from build123d import *

# Parameters (mm, degrees)
F3_R      = 4.5
F4_DEPTH  = 60.5
F8_DEPTH  = 60.5
F6_R      = 4.5
F6_R_2    = 4
F9_DEPTH  = 9.5
F7_R      = 4.5
F7_R_2    = 4
F10_DEPTH = 11
F11_R     = 2.5
F11_R_2   = 0.75
F12_DEPTH = 4.501


# Not quite as in the source:
# - ends of sketch curves that miss each other by under 0.0002 mm in the source are joined


with BuildPart() as f4:
    # F3 (on Front) → F4 (new body)
    with BuildSketch(Plane.XZ):
        Circle(F3_R)
    extrude(amount=F4_DEPTH)

    # F5 (on face) → F8 (cut, through all)
    with BuildSketch(Plane.XZ.offset(60.5)):
        with BuildLine():
            Line((-1.25, -3.8), (0, -3.8))
            Line((0, -3.8), (1.25, -3.8))
            Line((1.25, -3.8), (1.25, -3.7))
            ThreePointArc((1.25, -3.7), (1.3085786438, -3.5585786438), (1.45, -3.5))
            Line((1.45, -3.5), (2, -3.5))
            Line((2, -3.5), (2, -3.05))
            ThreePointArc((2, -3.05), (2.0585786438, -2.9085786438), (2.2, -2.85))
            Line((2.2, -2.85), (3.15, -2.85))
            Line((3.15, -2.85), (3.15, -2.15))
            Line((3.15, -2.15), (2.2, -2.15))
            ThreePointArc((2.2, -2.15), (2.0585786438, -2.0914213562), (2, -1.95))
            Line((2, -1.95), (2, -1.887459))
            ThreePointArc((2, -1.887459), (2.1033535752, -1.771554046), (2.2, -1.65))
            Line((2.2, -1.65), (3.75, -1.65))
            Line((3.75, -1.65), (3.75, 0))
            Line((3.75, 0), (3.75, 1.65))
            Line((3.75, 1.65), (2.2, 1.65))
            ThreePointArc((2.2, 1.65), (2.1033535752, 1.771554046), (1.9999998047, 1.8874588157))
            Line((1.9999998047, 1.8874588157), (2, 1.95))
            ThreePointArc((2, 1.95), (2.0585786438, 2.0914213562), (2.2, 2.15))
            Line((2.2, 2.15), (3.15, 2.15))
            Line((3.15, 2.15), (3.15, 2.85))
            Line((3.15, 2.85), (2.2, 2.85))
            ThreePointArc((2.2, 2.85), (2.0585786438, 2.9085786438), (2, 3.05))
            Line((2, 3.05), (2, 3.5))
            Line((2, 3.5), (1.45, 3.5))
            ThreePointArc((1.45, 3.5), (1.3085786438, 3.5585786438), (1.25, 3.7))
            Line((1.25, 3.7), (1.25, 3.8))
            Line((1.25, 3.8), (0, 3.8))
            Line((0, 3.8), (-1.25, 3.8))
            Line((-1.25, 3.8), (-1.25, 3.7))
            ThreePointArc((-1.25, 3.7), (-1.3085786438, 3.5585786438), (-1.45, 3.5))
            Line((-1.45, 3.5), (-2, 3.5))
            Line((-2, 3.5), (-2, 3.05))
            ThreePointArc((-2, 3.05), (-2.0585786438, 2.9085786438), (-2.2, 2.85))
            Line((-2.2, 2.85), (-3.15, 2.85))
            Line((-3.15, 2.85), (-3.15, 2.15))
            Line((-3.15, 2.15), (-2.2, 2.15))
            ThreePointArc((-2.2, 2.15), (-2.0585786438, 2.0914213562), (-2, 1.95))
            Line((-2, 1.95), (-2, 1.887459))
            ThreePointArc((-2, 1.887459), (-2.1033535752, 1.771554046), (-2.2, 1.65))
            Line((-2.2, 1.65), (-3.75, 1.65))
            Line((-3.75, 1.65), (-3.75, 0))
            Line((-3.75, 0), (-3.75, -1.65))
            Line((-3.75, -1.65), (-2.2, -1.65))
            ThreePointArc((-2.2, -1.65), (-2.1033535752, -1.771554046), (-1.9999998047, -1.8874588157))
            Line((-1.9999998047, -1.8874588157), (-2, -1.95))
            ThreePointArc((-2, -1.95), (-2.0585786438, -2.0914213562), (-2.2, -2.15))
            Line((-2.2, -2.15), (-3.15, -2.15))
            Line((-3.15, -2.15), (-3.15, -2.85))
            Line((-3.15, -2.85), (-2.2, -2.85))
            ThreePointArc((-2.2, -2.85), (-2.0585786438, -2.9085786438), (-2, -3.05))
            Line((-2, -3.05), (-2, -3.5))
            Line((-2, -3.5), (-1.45, -3.5))
            ThreePointArc((-1.45, -3.5), (-1.3085786438, -3.5585786438), (-1.25, -3.7))
            Line((-1.25, -3.7), (-1.25, -3.8))
        make_face()
    extrude(amount=-F8_DEPTH, mode=Mode.SUBTRACT)

    # F6 (on face) → F9 (join)
    with BuildSketch(Plane.XZ.offset(60.5)):
        Circle(F6_R)
        Circle(F6_R_2, mode=Mode.SUBTRACT)
    extrude(amount=F9_DEPTH)

    # F7 (on face) → F10 (join)
    with BuildSketch(Plane(origin=(0, 0, 0), x_dir=(-1, 0, 0), z_dir=(0, 1, 0))):
        Circle(F7_R)
        Circle(F7_R_2, mode=Mode.SUBTRACT)
    extrude(amount=F10_DEPTH)

    # F11 (on Right) → F12 (cut, through all)
    with BuildSketch(Plane.YZ):
        with Locations((-64, 0)):
            Circle(F11_R)
        with Locations((-68.25, 0)):
            Circle(F11_R_2)
    extrude(amount=-F12_DEPTH, mode=Mode.SUBTRACT)


solid = f4.part
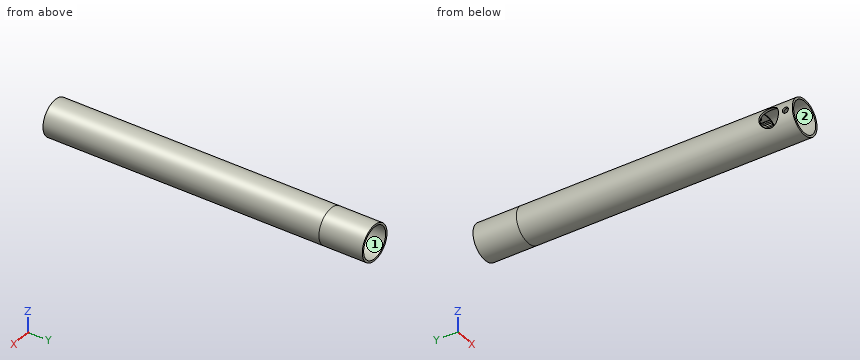
Read the model definition and answer for the solid it produces. Units are mm, in the model's axes. Face numbers are marked on the shaded views. A direction names the side the tool comes from. Give positions to 0.01 mm unless a question says otherwise; leave off trailing zeros. Loops run counter-clockwise (first coordinate to the right, second up) from the corner with the lowest first, then second, coordinate; pieces in that order, holes last. Notation, with made-up numbers: (47.25, 81.5) -> (98.25, 81.5) arc R15 cw to (98.25, 99.5) -> close; hole circle Ø3 at (-12.5, -11.5). An arc over 180 degrees is marked (long way). Use a Markdown table: item, result.
Q1. Section A-A, the plane x = 0 is taken. Determine the outline of the cut face in (y, z).
Solved:
| item | result |
|---|---|
| outline | (-70, -4.5) -> (11, -4.5) -> (11, -4) -> (0, -4) -> (0, -3.8) -> (-60.5, -3.8) -> (-60.5, -4) -> (-70, -4) -> close; (-70, 4) -> (-60.5, 4) -> (-60.5, 3.8) -> (0, 3.8) -> (0, 4) -> (11, 4) -> (11, 4.5) -> (-70, 4.5) -> close |
Q2. Each of these flat-tipped pins is pushed along its axis until it touches: pin 1 (0.9 mm diameter, centred on x = -2.5, z = -2, fed in from -Y); pin 2 (1 mm diameter, centred on x = -3, y = -20.5, fed in from -Z); pin 3 (0.8 mm diameter, centred on y = -18.5, z = 2.5, fed in from +X). Where does it stop, or does it pass through?
Solved:
| item | result |
|---|---|
| pin 1 | stops at y = -60.5 |
| pin 2 | stops at z = -3.74 |
| pin 3 | stops at x = 3.98 |
Q3. A tool of negligible diameter and unlimited length cuts with its end or side. For the marked faces 1 and 2, from which of +Z, -Z, +X, -X, +Y, -Y can it reach the whole face along a straight path? Write none if from no direction.
Solved:
| item | result |
|---|---|
| face 1 | +Y |
| face 2 | -Y |
Q4. Find the intervals of material crossed by line 1 along Z through (x, y) = (0, -65); line 2 along X through (y, z) = (-30, -3.75), in increasing order.
Solved:
| item | result |
|---|---|
| line 1 | z = -4.5 to -4, 4 to 4.5 |
| line 2 | x = -2.49 to -1.25, 1.25 to 2.49 |
Q5. Section B-B, the plane z = 0 is taken. Determine the outline of the cut face in (x, y), then the cut area to 3 significant figures.
Solved:
| item | result |
|---|---|
| outline | (-4.5, -70) -> (-4, -70) -> (-4, -69) -> (-4.5, -69) -> close; (-4.5, -67.5) -> (-4, -67.5) -> (-4, -66.5) -> (-4.5, -66.5) -> close; (-4.5, -61.5) -> (-4, -61.5) -> (-4, -60.5) -> (-3.75, -60.5) -> (-3.75, 0) -> (-4, 0) -> (-4, 11) -> (-4.5, 11) -> close; (3.75, -60.5) -> (4, -60.5) -> (4, -70) -> (4.5, -70) -> (4.5, 11) -> (4, 11) -> (4, 0) -> (3.75, 0) -> close |
| area | 108 mm^2 |
Q6. Section C-C, the plane y = -68.25 is taken. Determine the outline of the cut face in (x, z).
Solved:
| item | result |
|---|---|
| outline | (-4.44, -0.75) arc R4.5 ccw (long way) to (-4.44, 0.75) -> (-3.93, 0.75) arc R4 cw (long way) to (-3.93, -0.75) -> close |
